from build123d import *

# Parameters (mm, degrees)
F1_DEPTH = 63.5
F0_W     = 24.512149
F0_H     = 19.05
F2_DEPTH = 25.4
F3_DEPTH = 7.9375
F4_R     = 5.08


with BuildPart() as f1:
    # F0 (on Front) → F1 (new body, symmetric)
    with BuildSketch(Plane.XZ):
        Polygon((22.225, 9.525), (-41.275, 9.525), (-41.275, -9.525), (41.275, -9.525), (41.275, 9.525), align=None)
    extrude(amount=F1_DEPTH, both=True)

    # F0 (on Front) → F2 (join, symmetric)
    with BuildSketch(Plane.XZ):
        with BuildLine():
            Line((22.225, 26.3652), (22.225, 9.525))
            Line((22.225, 9.525), (41.275, 9.525))
            Line((41.275, 9.525), (41.275, 26.3652))
            ThreePointArc((41.275, 26.3652), (46.110667, 38.039533), (57.785, 42.8752))
            Line((57.785, 42.8752), (61.212851, 42.8752))
            Line((61.212851, 42.8752), (61.212851, 61.9252))
            Line((61.212851, 61.9252), (57.785, 61.9252))
            add(Edge.make_bspline(
                [(54.550323, 61.777775), (55.650758, 61.832388), (56.729755, 61.881267), (57.785, 61.9252)],
                knots=[108.765269, 108.765269, 108.765269, 108.765269, 112.065448, 112.065448, 112.065448, 112.065448], degree=3))
            ThreePointArc((54.550323, 61.777775), (31.521539, 50.339024), (22.225, 26.3652))
        make_face()
        with Locations((73.468925, 52.4002)):
            Rectangle(F0_W, F0_H)
    extrude(amount=F2_DEPTH, both=True)

    # F0 (on Front) → F3 (join, symmetric)
    with BuildSketch(Plane.XZ):
        with BuildLine():
            add(Edge.make_bspline(
                [(-41.275, 9.525), (-41.271032, 51.950031), (18.282835, 59.977869), (54.550323, 61.777775)],
                knots=[0, 0, 0, 0, 108.765269, 108.765269, 108.765269, 108.765269], degree=3))
            Line((-41.275, 9.525), (22.225, 9.525))
            Line((22.225, 9.525), (22.225, 26.3652))
            ThreePointArc((22.225, 26.3652), (31.521539, 50.339024), (54.550323, 61.777775))
        make_face()
    extrude(amount=F3_DEPTH, both=True)

    # F4
    f4_edges = [f1.edges().sort_by_distance(p)[0] for p in [
        (41.275, -63.5, 0),
        (41.275, 63.5, 0),
        (-41.275, -63.5, 0),
        (-41.275, 63.5, 0),
    ]]
    fillet(f4_edges, radius=F4_R)


solid = f1.part
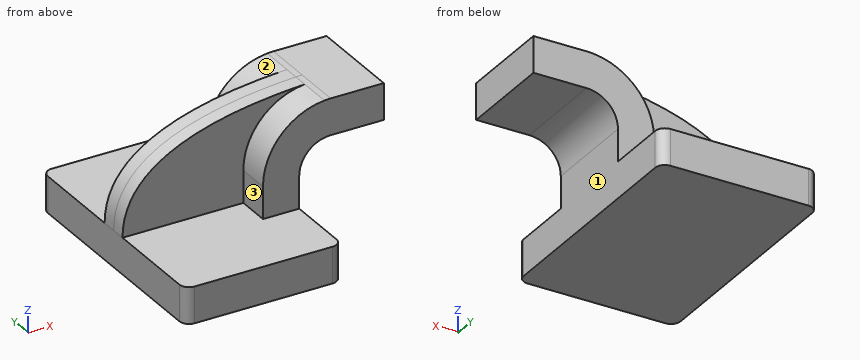
Model file for the job. Use its own axes, mm. Face numbers are marked on the shaded views. A direction names the side the tool comes from. Round coordinates to 2 decimals unless told otherwise and drop trailing zeros. Loops run counter-clockwise (first coordinate to the right, second up) from the corner with the lowest first, then second, coordinate; pieces in that order, holes last. Notation, with made-up numbers: (-11.75, 19) -> (36.25, 19) arc R32 cw to (36.25, 53) -> close; hole circle Ø3 at (60.5, 38). An arc over 180 degrees is marked (long way). Answer as CSV lines item,"result". Start each with the question number.
1) Slice it at A-A (z = 7). List the corners of the cut face in (x, y) (3 decimals).
2) Probe line 1 along Z through (x, y) = (5.5, 32) (3 decimals); line 2 along X through (y, z) = (53, 8.5) (3 decimals); line 3 along Y through (x, z) = (-25, 35). List the from-to ranges inside material, lowest first.
3) Slice it at C-C (y = -39). List the corners of the cut face in (x, z) (3 decimals).
4) Slice it at B-B (x = 72). List the corners of the cut face in (y, z), plus the area to 3 significant figures.
5) Tool access for the marked faces 1, 2 and 3: list every direction of +Z, -Z, +X, -X, +Y, -Y with a clear straight run to the whole face (end or side of a thin tool).
6) Pin check, flat tips, straight feed: P1, Ø8, axis at x = -0.5, z = 33.5, coming from the +Y side; P2, Ø15.5, axis at x = 63.5, z = 28.5, coming from the -Y side; P3, Ø18.5, axis at y = -14, z = 15.5, coming from the -X side (3 decimals); P4, Ø11, axis at y = 20, z = 5.5, coming from the +X side (3 decimals). Stop position of each tip, or through.
Filled in:
1,outline,"(-41.275, -58.42) arc R5.08 ccw to (-36.195, -63.5) -> (36.195, -63.5) arc R5.08 ccw to (41.275, -58.42) -> (41.275, 58.42) arc R5.08 ccw to (36.195, 63.5) -> (-36.195, 63.5) arc R5.08 ccw to (-41.275, 58.42) -> close"
2,line 1,"z = -9.525 to 9.525"
2,line 2,"x = -41.275 to 41.275"
2,line 3,"y = -7.94 to 7.94"
3,outline,"(-41.275, -9.525) -> (41.275, -9.525) -> (41.275, 9.525) -> (-41.275, 9.525) -> close"
4,outline,"(-25.4, 42.88) -> (25.4, 42.88) -> (25.4, 61.93) -> (-25.4, 61.93) -> close"
4,area,"968 mm2"
5,face 1,"-Z, +X, +Y, -Y"
5,face 2,"+Z, -X, +Y"
5,face 3,"+Z, -X, -Y"
6,P1,"stops at y = 7.94"
6,P2,"passes through"
6,P3,"stops at x = -41.275"
6,P4,"stops at x = 41.275"
